Autodesk Inventor part; units mm, degrees
ref_plane "YZ Plane" through (0, 0, 0) normal (1, 0, 0) x (0, 1, 0)
ref_plane "XZ Plane" through (0, 0, 0) normal (0, 1, 0) x (-1, 0, 0)
ref_plane "XY Plane" through (0, 0, 0) normal (0, 0, 1) x (1, 0, 0)
sketch "Sketch1" plane through (0, 0, 0) normal (0, 1, 0) x (-1, 0, 0)
  line L0 (0, 0) -> (2, 0) construction
  line L1 (0, -75) -> (2, -75) construction
  line L2 (0, -73) -> (2.4733, -73)
  line L3 (1.3383, -13) -> (1.3383, -5.3327) construction
  line L4 (6.5938, -37.5) -> (0, -37.5) construction
  line L5 (2.0086, -8.9832) -> (-0.0001, -8.9832) construction
  arc A0 (0.4733, -73) -> (-2.5001, -8.9832) centre (-105.0089, -45.8218) ccw
  arc A1 (2.4733, -73) -> (-0.5001, -8.9832) centre (-103.0089, -45.8218) ccw
  line L6 (-0.5001, -8.9832) -> (-2.5001, -8.9832)
  line L7 (-0.9649, -13.5728) -> (-5.9649, -13.5728)
  line L8 (-5.9649, -13.5728) -> (-5.9649, -10.8228)
  line L9 (-5.9649, -10.8228) -> (-1.8575, -10.8228)
  line L10 (-3.6617, -68.25) -> (-8.7098, -68.25) construction
  line L11 (1.5844, -68.25) -> (-5.9649, -68.25)
  line L12 (-5.9649, -68.25) -> (-5.9649, -71)
  line L13 (-5.9649, -71) -> (0.9685, -71)
  line L14 (-5.9649, -13.5728) -> (-5.9649, -68.25)
  line L15 (-0.9649, -13.5728) -> (-0.9649, -15.2728)
  line L16 (-0.9649, -66.55) -> (1.9279, -66.55)
  line L17 (3.9279, -66.55) -> (1.9279, -66.55)
  line L18 (-0.9649, -15.2728) -> (-0.4532, -15.2728)
  line L19 (1.5468, -15.2728) -> (-0.4532, -15.2728)
  line L20 (-0.9649, -15.2728) -> (-0.9649, -66.55)
  line L21 (-0.9649, -66.55) -> (-0.9649, -68.25)
  point P0 (0.0167, -6.9833)
  point P1 (2, 0)
  point P2 (4.5938, -37.5)
  point P3 (0, -41)
  point P4 (0, -15)
  point P5 (0, -67.5)
  point P6 (0, -69)
  point P7 (0, -13)
  point P8 (3.8363, -67.0175)
  point P9 (-3.6617, -13.5728)
  point P10 (0.9193, -71)
  point P11 (1.5637, -68.25)
  point P12 (2.3337, -10.8228)
  point P13 (-3.6617, -10.8228)
  point P14 (1.3383, -13.5728)
  point P15 (3.6, -37.5)
  point P16 (5.6, -37.5)
  point P17 (-0.5333, -15)
  point P18 (1.4667, -15)
  dimension "d1" = 2
  dimension "d3" = 2
  dimension "d4" = 2
  dimension "d5" = 2
  dimension "d6" = 32
  dimension "d8" = 3.6
  dimension "d9" = 2
  dimension "d10" = 2.5
  dimension "d11" = 2
  dimension "d12" = 5
  dimension "d29" = 1.7
extrude "Extrusion12" add sketch "Sketch1" along normal blind 138 contours A0 L17 A1 L2 | L17 A0 L19 A1 | L19 A0 L6 A1
extrude "Extrusion13" add sketch "Sketch1" along normal blind 133 contours L13 L12 L11 A0 | L11 L21 L16 A0 | L16 L20 L18 A0 | L11 L14 L7 L15 L20 L21 | L18 L15 A0 | L8 L9 A0 L7
extrude "Extrusion14" cut sketch "Sketch1" along normal blind 129 contours L17 A0 L19 A1
extrude "Extrusion15" cut sketch "Sketch1" along normal blind 131 contours L11 L14 L7 L15 L20 L21
extrude "Extrusion16" cut sketch "Sketch1" along normal blind 129 contours L16 L20 L18 A0
extrude "Extrusion17" add sketch "Sketch1" along normal blind 51 contours L17 A0 L19 A1 | L16 L20 L18 A0
extrude "Extrusion18" add sketch "Sketch1" along normal blind 46 contours L11 L14 L7 L15 L20 L21
extrude "Extrusion20" cut sketch "Sketch1" along normal blind 43 contours L13 L12 L11 A0 | L11 L21 L16 A0 | L16 L20 L18 A0 | L11 L14 L7 L15 L20 L21 | L18 L15 A0 | L8 L9 A0 L7
properties part number "face_v3"
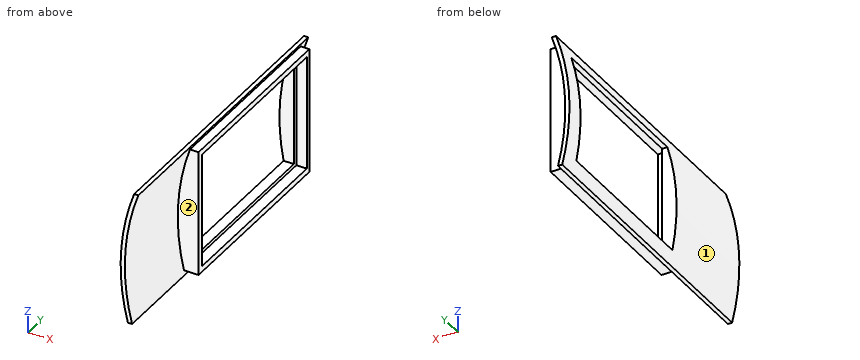
CAD build for the part. Positions are in the model's coordinates, mm. Face numbers are marked on the shaded views. A direction names the side the tool comes from. Give positions to 0.01 mm unless a question says otherwise; leave off trailing zeros. Order: outer loops, then holes, each group sorted by start corner. A loop starts at its lowest first (then second) coordinate and runs counter-clockwise, first axis right, second up. Notation, with made-up numbers: (50, 83) - (104, 83) arc R27 cw to (104, 104) - close; hole circle Ø4 at (-34, 6.5). An arc over 180 degrees is marked (long way). Write each question's results on one line, items separated by ' | '.
1. Pin check, flat tips, straight feed: pin 1 (4.5 mm diameter, centred on x = 5, y = 91, fed in from +Z); pin 2 (3 mm diameter, centred on x = 4.5, y = 36, fed in from -Z); pin 3 (1.5 mm diameter, centred on x = 2, z = -19.5, fed in from -Y); pin 4 (5.5 mm diameter, centred on x = 4.5, y = 101.5, fed in from -Z). Stop position of each tip, or through.
Calculated:
pin 1: stops at z = -10.82 | pin 2: passes through | pin 3: stops at y = 43 | pin 4: stops at z = -71
2. 3-axis set-ups, long thin cutter, end or side, ignore diameter. For the marked faces 1 and 2: which of +Z, -Z, +X, -X, +Y, -Y reach the whole face in a straight line?
Calculated:
face 1: -X, +Y, -Y | face 2: +X, -Y
3. Saw through at C-C on x = 4.5. List the corners of the cut face in (y, z).
Calculated:
outline: (43, -71) - (133, -71) - (133, -10.82) - (43, -10.82) - close; hole (46, -68.25) - (131, -68.25) - (131, -13.57) - (46, -13.57) - close
4. Probe L1, parallel to Y at x = 5.25, z = -34; L2, parallel to Y at x = -1.75, z = -65; L3, parallel to Z at x = 4, y = 110. List the from-to ranges inside material, lowest first. Write a range as from..to.
Calculated:
L1: y = 43..46, 131..133 | L2: y = 43..51, 129..133 | L3: z = -71..-68.25, -13.57..-10.82
5. Saw through at B-B on y = 66.5. List the corners of the cut face in (x, z).
Calculated:
outline: (-3.93, -66.55) arc R108.93 ccw to (-2.47, -73) - (-0.47, -73) arc R108.93 cw to (-0.97, -71) - (5.96, -71) - (5.96, -68.25) - (0.96, -68.25) - (0.96, -66.55) - close; (-1.55, -15.27) - (0.96, -15.27) - (0.96, -13.57) - (5.96, -13.57) - (5.96, -10.82) - (1.86, -10.82) arc R108.93 cw to (2.5, -8.98) - (0.5, -8.98) arc R108.93 ccw to start
6. Saw through at A-A on z = -39.5. List the corners of the cut face in (x, y).
Calculated:
outline: (-5.73, 0) - (-3.73, 0) - (-3.73, 43) - (5.96, 43) - (5.96, 46) - (0.96, 46) - (0.96, 51) - (-5.73, 51) - close; (-5.73, 129) - (0.96, 129) - (0.96, 131) - (5.96, 131) - (5.96, 133) - (-3.73, 133) - (-3.73, 138) - (-5.73, 138) - close
7. Saw through at D-D on y = 12. List the corners of the cut face in (x, z), and give its area (3 significant figures).
Calculated:
outline: (-2.47, -73) - (-0.47, -73) arc R108.93 cw to (2.5, -8.98) - (0.5, -8.98) arc R108.93 ccw to start | area: 128 mm2
